Study the drawing (mm; zero at the part's minimum x, y, z) and answer. Coordinates: 2 decimals unless noted, no trailing zeros. Write each loop counter-clockwise with the first axis right and the second up, starting at its lowest first coordinate (ties: lowest second). Pieces come first, ordered by that corner, then holes. Notation, with made-up numbers: M 15,81.25 L 68,81.25 A23 ccw 68,100.25 Z; hole C -32.75,51.5 d1. An arc over 180 degrees is marked long. Answer as CSV lines item,"result". Start each with the question number.
(1) Flat-ended cylindrical pins translate along their axes: P1, Ø2, axis at y = 15.5, z = 53.5, coming from the +X side; P2, Ø1, axis at x = 13.5, z = 59, coming from the +Y side; P3, Ø2, axis at y = 13.5, z = 102.5, coming from the +X side; P4, Ø5, axis at y = 10, z = 9.45, coming from the -X side. Find the tip coordinate at first contact, or state that the pin passes through.
(2) A cutting plane is placed at B-B on x = 3. Give the vertices of the cut face in (y, z).
(3) A cutting plane is placed at C-C on z = 95. Give the vertices of the cut face in (x, y).
(4) A cutting plane is placed at A-A on y = 10. Give the vertices of the cut face in (x, z).
(5) A cutting plane is placed at D-D on z = 9.45. Give the vertices of the cut face in (x, y).
(6) Find the intervals of material crossed by L1, parallel to Z at x = 7, y = 10; L2, parallel to Z at x = 15, y = 9; L3, parallel to X at y = 9.5, z = 13, in increasing order. Write a range as [from, to].
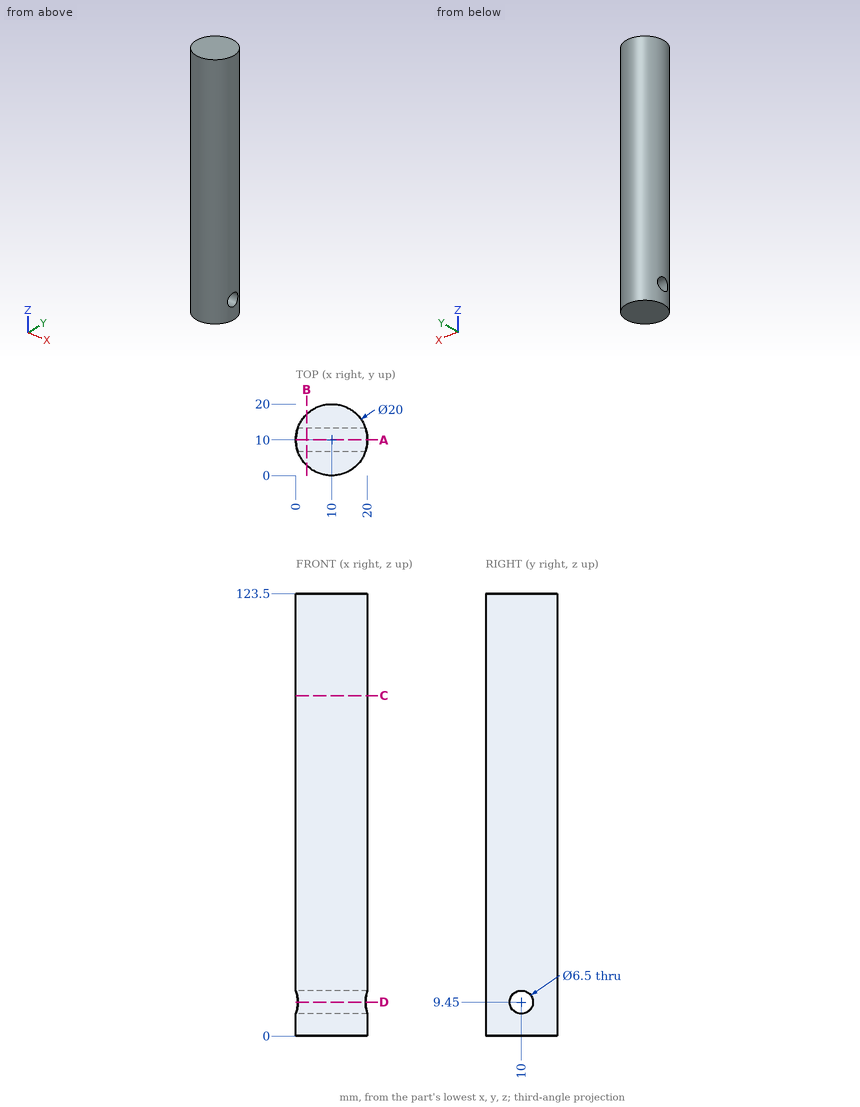
Here are the results:
1,P1,"stops at x = 18.93"
1,P2,"stops at y = 19.54"
1,P3,"stops at x = 19.68"
1,P4,"passes through"
2,outline,"M 2.86,0 L 17.14,0 L 17.14,123.5 L 2.86,123.5 Z; hole C 10,9.45 d6.5"
3,outline,"C 10,10 d20"
4,outline,"M 0,0 L 20,0 L 20,6.2 L 0,6.2 Z; M 0,12.7 L 20,12.7 L 20,123.5 L 0,123.5 Z"
5,outline,"M 0.54,6.75 A10 ccw 19.46,6.75 Z; M 0.54,13.25 L 19.46,13.25 A10 ccw Z"
6,L1,"z = [0, 6.2], [12.7, 123.5]"
6,L2,"z = [0, 6.36], [12.54, 123.5]"
6,L3,"x = [0.01, 19.99]"
